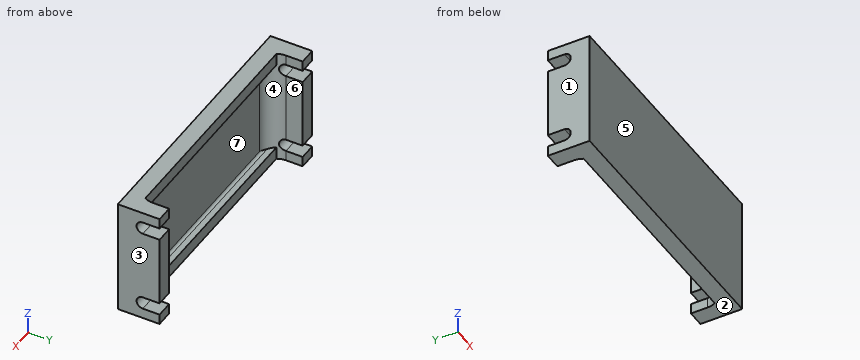
from build123d import *

# Parameters (mm, degrees)
SKETCH1_W           = 101.6
SKETCH1_H           = 44.45
BOSS_EXTRUDE1_DEPTH = 3.175
SKETCH2_W           = 6.35
SKETCH2_H           = 44.45
BOSS_EXTRUDE2_DEPTH = 12.7
SKETCH3_W           = 88.9
SKETCH3_H           = 4.7625
BOSS_EXTRUDE3_DEPTH = 3.175
FILLET1_R           = 0.9525
FILLET2_R           = 6.35
SKETCH4_R           = 2.38125
CUT_EXTRUDE1_DEPTH  = 106.20706371


with BuildPart() as part:
    # Sketch1 → Boss-Extrude1 (new body)
    with BuildSketch(Plane(origin=(0, 0, 0), x_dir=(1, 0, 0), z_dir=(0, 1, 0))):
        Rectangle(SKETCH1_W, SKETCH1_H)
    extrude(amount=BOSS_EXTRUDE1_DEPTH)

    # Sketch2 → Boss-Extrude2 (add)
    with BuildSketch(Plane(origin=(0, 3.175, 0), x_dir=(1, 0, 0), z_dir=(0, 1, 0))):
        with Locations((-47.625, 0)):
            Rectangle(SKETCH2_W, SKETCH2_H)
        with Locations((47.625, 0)):
            Rectangle(SKETCH2_W, SKETCH2_H)
    extrude(amount=BOSS_EXTRUDE2_DEPTH)

    # Sketch3 → Boss-Extrude3 (add)
    with BuildSketch(Plane(origin=(0, 3.175, 0), x_dir=(1, 0, 0), z_dir=(0, 1, 0))):
        with Locations((0, 19.84375)):
            Rectangle(SKETCH3_W, SKETCH3_H)
        with Locations((0, -19.84375)):
            Rectangle(SKETCH3_W, SKETCH3_H)
    extrude(amount=BOSS_EXTRUDE3_DEPTH)

    # Fillet1
    fillet1_edges = [part.edges().sort_by_distance(p)[0] for p in [
        (0, 3.175, 17.4625),
        (0, 3.175, -17.4625),
    ]]
    fillet(fillet1_edges, radius=FILLET1_R)

    # Fillet2
    # the kernel refuses this fillet: 6.35 mm, written as the material it adds along each edge
    with BuildSketch(Plane(origin=(44.45, 3.175, -32.385), x_dir=(0, 1, 0), z_dir=(0, 0, 1))) as fillet2_piece_1_section:
        with BuildLine():
            CenterArc((FILLET2_R, FILLET2_R), FILLET2_R, 180, 90)
            Line((0, FILLET2_R), (0, 0))
            Line((0, 0), (FILLET2_R, 0))
        make_face()
    fillet2_piece_1 = extrude(amount=64.77, mode=Mode.PRIVATE)
    fillet2_piece_1 = split(fillet2_piece_1, bisect_by=Plane(origin=(44.198002836, 7.13272394, -22.225), z_dir=(0, 0, 1)), keep=Keep.TOP, mode=Mode.PRIVATE)
    fillet2_piece_1 = split(fillet2_piece_1, bisect_by=Plane(origin=(44.198002836, 7.13272394, 22.225), z_dir=(0, 0, -1)), keep=Keep.TOP, mode=Mode.PRIVATE)
    add(fillet2_piece_1)
    with BuildSketch(Plane(origin=(-44.45, 3.175, -32.385), x_dir=(1, 0, 0), z_dir=(0, 0, 1))) as fillet2_piece_2_section:
        with BuildLine():
            CenterArc((FILLET2_R, FILLET2_R), FILLET2_R, 180, 90)
            Line((0, FILLET2_R), (0, 0))
            Line((0, 0), (FILLET2_R, 0))
        make_face()
    fillet2_piece_2 = extrude(amount=64.77, mode=Mode.PRIVATE)
    fillet2_piece_2 = split(fillet2_piece_2, bisect_by=Plane(origin=(-44.198002836, 7.13272394, -22.225), z_dir=(0, 0, 1)), keep=Keep.TOP, mode=Mode.PRIVATE)
    fillet2_piece_2 = split(fillet2_piece_2, bisect_by=Plane(origin=(-44.198002836, 7.13272394, 22.225), z_dir=(0, 0, -1)), keep=Keep.TOP, mode=Mode.PRIVATE)
    add(fillet2_piece_2)

    # Sketch4 → Cut-Extrude1 (cut, through all)
    with BuildSketch(Plane(origin=(50.8, 0, 0), x_dir=(0, 0, -1), z_dir=(1, 0, 0))):
        with BuildLine():
            Line((-18.25625, 15.875), (-18.25625, 9.525))
            ThreePointArc((-18.25625, 9.525), (-15.875, 11.90625), (-13.49375, 9.525))
            Line((-13.49375, 9.525), (-13.49375, 15.875))
            Line((-13.49375, 15.875), (-18.25625, 15.875))
        make_face()
        with Locations((-15.875, 9.525)):
            Circle(SKETCH4_R)
        with Locations((15.875, 9.525)):
            Circle(SKETCH4_R)
        with BuildLine():
            Line((18.25625, 15.875), (13.49375, 15.875))
            Line((13.49375, 15.875), (13.49375, 9.525))
            ThreePointArc((13.49375, 9.525), (15.875, 11.90625), (18.25625, 9.525))
            Line((18.25625, 9.525), (18.25625, 15.875))
        make_face()
    extrude(amount=-CUT_EXTRUDE1_DEPTH, mode=Mode.SUBTRACT)


solid = part.part
Verification items for the finished model (mm, model axes). Face numbers are marked on the shaded views. A direction names the side the tool comes from. Give positions to 0.01 mm unless a question says otherwise; leave off trailing zeros. Write each loop counter-clockwise with the first axis right and the second up, starting at its lowest first coordinate (ties: lowest second). Pieces come first, ordered by that corner, then holes. Notation, with made-up numbers: M 1,-35 L 38,-35 A11 ccw 38,-18 Z; hole C 26,27 d8. An arc over 180 degrees is marked long. Put each result on its own line as item: value. Start each with the question number.
1. Go/stop test with flat-tipped pins: pin 1 Ø4 at (x, z) = (4.5, -19) entering from +Y; pin 2 Ø8 at (x, y) = (-5, 9) entering from +Z (3 decimals); pin 3 Ø10 at (x, z) = (-10, -1.5) entering from +Y (3 decimals). Record where each tip stops, or that it passes through.
2. Section check D-D (y = 5.25). Record the cut outline in (x, z) (1 decimal), and give its area (3 significant figures).
3. Set-up check for the marked faces 5, 6 and 7: record each of +Z, -Z, +X, -X, +Y, -Y from which the full face is reachable in a straight line by a thin tool's end or side.
4. Section check A-A (y = 14). Record the cut outline in (x, z) (3 decimals), and give its area (3 significant figures).
5. Section check B-B (z = 10). Record the cut outline in (x, y) (3 decimals), and give its area (3 significant figures).
6. Draft check along X on the marked faces 1, 2, 3 and 4. Enter one of: +X half, -X half, draft (parallel to the pull), parting line (faces both ways), or undercut.
7. Scan lines: line 1 along X through (y, z) = (13.25, -20); line 2 along Z through (x, y) = (0.5, 5.25) (1 decimal); line 3 along Y through (x, z) = (-5, 12.5) (3 decimals). Record each from-to range of solid material in increasing order. Write a range as [from, to].
Answer list:
1. pin 1: y = 6.35
1. pin 2: z = 22.225
1. pin 3: y = 3.175
2. outline: M -50.8,-22.2 L 50.8,-22.2 L 50.8,22.2 L -50.8,22.2 Z; hole M -42.8,-17.5 L 42.8,-17.5 L 42.8,17.5 L -42.8,17.5 Z
2. area: 1,530 mm2
3. face 5: +Z, -Z, +X, -X, -Y
3. face 6: +Z, -Z, +Y
3. face 7: +Y
4. outline: M -50.8,-22.225 L -44.45,-22.225 L -44.45,-18.256 L -50.8,-18.256 Z; M -50.8,-13.494 L -44.45,-13.494 L -44.45,13.494 L -50.8,13.494 Z; M -50.8,18.256 L -44.45,18.256 L -44.45,22.225 L -50.8,22.225 Z; M 44.45,-22.225 L 50.8,-22.225 L 50.8,-18.256 L 44.45,-18.256 Z; M 44.45,-13.494 L 50.8,-13.494 L 50.8,13.494 L 44.45,13.494 Z; M 44.45,18.256 L 50.8,18.256 L 50.8,22.225 L 44.45,22.225 Z
4. area: 444 mm2
5. outline: M -50.8,0 L 50.8,0 L 50.8,15.875 L 44.45,15.875 L 44.45,9.525 A6.35 cw 38.1,3.175 L -38.1,3.175 A6.35 cw -44.45,9.525 L -44.45,15.875 L -50.8,15.875 Z
5. area: 501 mm2
6. face 1: -X half
6. face 2: draft
6. face 3: +X half
6. face 4: undercut
7. line 1: [-50.8, -44.45], [44.45, 50.8]
7. line 2: [-22.2, -17.5], [17.5, 22.2]
7. line 3: [0, 3.175]
